Read the model definition and answer for the solid it produces. Units are mm, in the model's axes. Coordinates: 2 decimals unless noted, no trailing zeros. Loops run counter-clockwise (first coordinate to the right, second up) from the corner with the lowest first, then second, coordinate; pieces in that order, holes last. Notation, with made-up numbers: M 67,82.25 L 109,82.25 A17 ccw 109,98.25 Z; hole C 31.25,88 d5. An arc over 180 degrees is marked long. One line per item, written item: value. Start each with the question number.
1. The part is cut by section A-A (y = 1.35). Write down the section's boundary in (x, z), then the cut area to 3 significant figures.
2. Consider probe 1 along X at (y, z) = (0.9, -1.8); probe 2 along X at (y, z) = (0.8, 1.3); probe 3 along Z at (x, y) = (3, 1.9). Determine where each line is inside the solid, lowest interval first.
3. The part is cut by section B-B (z = -0.25). Write down the section's boundary in (x, y).
4. The part is cut by section C-C (x = 2). Write down the section's boundary in (y, z), then the cut area to 3 significant figures.
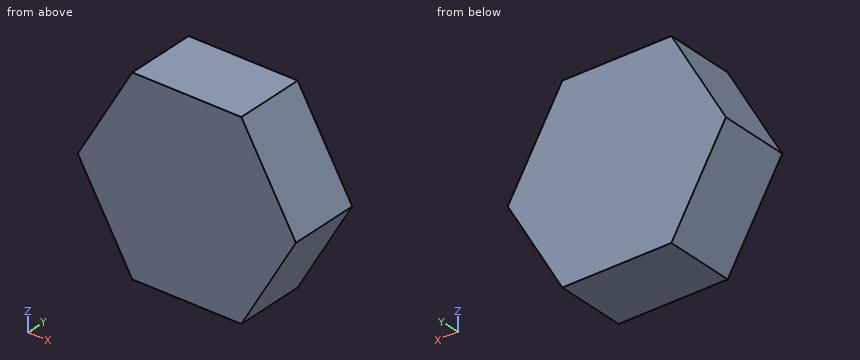
Autodesk Fusion 360 part; units mm, degrees
sketch "Sketch1" plane through (0, 0, 0) normal (0, 1, 0) x (1, 0, 0)
  line L0 (-1.7321, -3) -> (1.7321, -3)
  line L1 (1.7321, -3) -> (3.4641, 0)
  line L2 (3.4641, 0) -> (1.7321, 3)
  line L3 (1.7321, 3) -> (-1.7321, 3)
  line L4 (-1.7321, 3) -> (-3.4641, 0)
  line L5 (-3.4641, 0) -> (-1.7321, -3)
  line L6 (-1.7321, -3) -> (1.7321, 3)
  line L7 (-1.7321, 3) -> (1.7321, -3)
  line L8 (3.4641, 0) -> (-3.4641, 0)
  dimension "d1" = 120
  dimension "d2" = 120
  dimension "d3" = 6
  dimension "d4" = 6
  dimension "d5" = 6
extrude "Extrude1" add sketch "Sketch1" along normal blind 2.25
equation "d3 = d4"
equation "d5 = d4"
Answer block:
1. outline: M -3.46,0 L -1.73,-3 L 1.73,-3 L 3.46,0 L 1.73,3 L -1.73,3 Z
1. area: 31.2 mm2
2. probe 1: x = -2.42 to 2.42
2. probe 2: x = -2.71 to 2.71
2. probe 3: z = -0.8 to 0.8
3. outline: M -3.32,0 L 3.32,0 L 3.32,2.25 L -3.32,2.25 Z
4. outline: M 0,-2.54 L 2.25,-2.54 L 2.25,2.54 L 0,2.54 Z
4. area: 11.4 mm2
